The model under review builds one solid part; all positions refer to its coordinate system, in mm. Face numbers are marked on the shaded views. A direction names the side the tool comes from. Round coordinates to 2 decimals unless told otherwise and drop trailing zeros. Write each loop counter-clockwise with the first axis right and the second up, starting at its lowest first coordinate (ties: lowest second). Pieces come first, ordered by that corner, then holes.
Item 1: Draft analysis for pull direction Z (two halves, no side actions). For the marked faces 3, 4, 5 and 6, state which applies: +Z half, -Z half, draft (parallel to the pull), parting line (faces both ways), or undercut.
Item 2: Add section B-B (x = 10.5). Give the boundary of the cut face in (y, z) (3 decimals), plus the area to 3 significant figures.
Item 3: Machinability: for the marked faces 1 and 2, which of the approach directions +Z, -Z, +X, -X, +Y, -Y give a long, thin tool a straight path to every point of the face, cutting with its end or side? Answer none if there is none.
Item 4: To check wall thickness, follow L1, parallel to X at y = -3.5, z = 36.83; L2, parallel to X at y = 19.5, z = 33; L3, parallel to X at y = 8, z = 36.83. State the ranges of each line that lie inside material, in increasing order.
Item 5: Add section A-A (z = -36.83). Give the boundary of the cut face in (x, y) (3 decimals), plus the area to 3 significant figures.
Item 6: Add section D-D (y = -3.5). Give the boundary of the cut face in (x, z).
Item 7: Clearance check with flat-ended pins moving along their axes: pin 1 Ø2 at (x, z) = (28.5, 1.5) entering from +Y; pin 2 Ø8 at (x, z) = (17, 7.5) entering from -Y; pin 3 Ø5.5 at (x, y) = (-18, 8.5) entering from +Z (3 decimals); pin 4 Ø1.5 at (y, z) = (7.5, 14.5) entering from +X. State where each tip first meets the part, or that it passes through.
Item 8: Add section C-C (z = -8). State how many separate pieces and enclosed holes the cut face has, plus the area to 3 significant figures.
```python
from build123d import *

# Parameters (mm, degrees)
SKETCH1_W           = 103.124
SKETCH1_H           = 80.01
SKETCH1_W_2         = 90.424
SKETCH1_H_2         = 70.612
BOSS_EXTRUDE3_DEPTH = 21.59
SKETCH1_4_W         = 90.424
SKETCH1_4_H         = 70.612
SKETCH1_4_R         = 1.27
SKETCH1_4_W_2       = 6.35
SKETCH1_4_H_2       = 38.1
BOSS_EXTRUDE4_DEPTH = 2.54
SKETCH2_W           = 16.256
SKETCH2_H           = 14.732
SKETCH2_W_2         = 13.208
SKETCH2_H_2         = 16.51
CUT_EXTRUDE1_DEPTH  = 6.35
SKETCH6_W           = 65.024
SKETCH6_H           = 9.525
CUT_EXTRUDE2_DEPTH  = 3.048
SKETCH8_R           = 2.393
SKETCH8_R_2         = 1.25
BOSS_EXTRUDE5_DEPTH = 6.35


# Read off the part's stored shape, not the designer's step: Ø2.5mm Dowel Hole1
with BuildPart() as part:
    # Sketch1 → Boss-Extrude3 (new body)
    with BuildSketch(Plane(origin=(0, 0, 0), x_dir=(1, 0, 0), z_dir=(0, 1, 0))):
        Rectangle(SKETCH1_W, SKETCH1_H)
        with Locations((0, -1.651)):
            Rectangle(SKETCH1_W_2, SKETCH1_H_2, mode=Mode.SUBTRACT)
    extrude(amount=BOSS_EXTRUDE3_DEPTH)

    # Sketch1<4> → Boss-Extrude4 (add)
    with BuildSketch(Plane(origin=(0, 0, 0), x_dir=(1, 0, 0), z_dir=(0, 1, 0))):
        with Locations((0, -1.651)):
            Rectangle(SKETCH1_4_W, SKETCH1_4_H)
        with Locations(Location((-40.024126951, -20.193, 0), (0, 0, 270))):
            Circle(SKETCH1_4_R, mode=Mode.SUBTRACT)
        with Locations((-30.48, 0)):
            Rectangle(SKETCH1_4_W_2, SKETCH1_4_H_2, mode=Mode.SUBTRACT)
        with Locations((-15.24, 0)):
            Rectangle(SKETCH1_4_W_2, SKETCH1_4_H_2, mode=Mode.SUBTRACT)
        Rectangle(SKETCH1_4_W_2, SKETCH1_4_H_2, mode=Mode.SUBTRACT)
        with BuildLine():
            ThreePointArc((18.415, -19.037561911), (18.956131264, -19.506178054), (19.157873049, -20.193))
            ThreePointArc((19.157873049, -20.193), (16.819614834, -20.879821946), (18.415, -19.037561911))
        make_face(mode=Mode.SUBTRACT)
        Polygon((12.065, -19.05), (12.065, 19.05), (18.415, 19.05), (18.415, -13.196681286), (15.24, -13.196681286), (15.24, -19.05), align=None, mode=Mode.SUBTRACT)
        with Locations((30.48, 0)):
            Rectangle(SKETCH1_4_W_2, SKETCH1_4_H_2, mode=Mode.SUBTRACT)
        with Locations(Location((-40.024126951, 28.575, 0), (0, 0, 270))):
            Circle(SKETCH1_4_R, mode=Mode.SUBTRACT)
        with Locations(Location((17.887873049, 28.575, 0), (0, 0, 270))):
            Circle(SKETCH1_4_R, mode=Mode.SUBTRACT)
    extrude(amount=BOSS_EXTRUDE4_DEPTH)

    # Sketch2 → Cut-Extrude1 (cut)
    with BuildSketch(Plane(origin=(51.562, 0, 0), x_dir=(0, 0, -1), z_dir=(1, 0, 0))):
        with Locations((-12.827, 9.906)):
            Rectangle(SKETCH2_W, SKETCH2_H)
        with Locations((5.715, 10.795)):
            Rectangle(SKETCH2_W_2, SKETCH2_H_2)
        with Locations((23.241, 10.795)):
            Rectangle(SKETCH2_W_2, SKETCH2_H_2)
    extrude(amount=-CUT_EXTRUDE1_DEPTH, mode=Mode.SUBTRACT)

    # Ø2.5mm Dowel Hole1 outline → Ø2.5mm Dowel Hole1 (revolve, cut)
    with BuildSketch(Plane(origin=(48.387, 0, -36.83), x_dir=(1, 0, 0), z_dir=(0, 0, 1))):
        Polygon((0, 0), (1.25, 0), (1.25, 21.565), (1.275, 21.59), (0, 21.59), align=None)
    revolve(axis=Axis((48.387, 0, -36.83), (0, 1, 0)), mode=Mode.SUBTRACT)

    # 2.5mm Dowel Hole1 2 outline → 2.5mm Dowel Hole1 2 (revolve, cut)
    with BuildSketch(Plane(origin=(48.387, 0, 36.83), x_dir=(1, 0, 0), z_dir=(0, 0, 1))):
        Polygon((0, 0), (1.25, 0), (1.25, 21.565), (1.275, 21.59), (0, 21.59), align=None)
    revolve(axis=Axis((48.387, 0, 36.83), (0, 1, 0)), mode=Mode.SUBTRACT)

    # 2.5mm Dowel Hole1 3 outline → 2.5mm Dowel Hole1 3 (revolve, cut)
    with BuildSketch(Plane(origin=(-48.387, 0, -36.83), x_dir=(1, 0, 0), z_dir=(0, 0, 1))):
        Polygon((0, 0), (1.25, 0), (1.25, 21.565), (1.275, 21.59), (0, 21.59), align=None)
    revolve(axis=Axis((-48.387, 0, -36.83), (0, 1, 0)), mode=Mode.SUBTRACT)

    # 2.5mm Dowel Hole1 4 outline → 2.5mm Dowel Hole1 4 (revolve, cut)
    with BuildSketch(Plane(origin=(-48.387, 0, 36.83), x_dir=(1, 0, 0), z_dir=(0, 0, 1))):
        Polygon((0, 0), (1.25, 0), (1.25, 21.565), (1.275, 21.59), (0, 21.59), align=None)
    revolve(axis=Axis((-48.387, 0, 36.83), (0, 1, 0)), mode=Mode.SUBTRACT)

    # Sketch6 → Cut-Extrude2 (cut)
    with BuildSketch(Plane.XY.offset(40.005)):
        with Locations((-12.7, 7.9375)):
            Rectangle(SKETCH6_W, SKETCH6_H)
    extrude(amount=-CUT_EXTRUDE2_DEPTH, mode=Mode.SUBTRACT)

    # Sketch8 → Boss-Extrude5 (add)
    # profile 1 of 4: a face of its own
    with BuildSketch(Plane.XZ):
        with Locations(Location((-48.387, 36.83, 0), (0, 0, 90))):
            Circle(SKETCH8_R)
        with Locations(Location((-48.387, 36.83, 0), (0, 0, 90))):
            Circle(SKETCH8_R_2, mode=Mode.SUBTRACT)
    # profile 2 of 4: a face of its own
    with BuildSketch(Plane.XZ):
        with Locations(Location((48.387, 36.83, 0), (0, 0, 270))):
            Circle(SKETCH8_R)
        with Locations(Location((48.387, 36.83, 0), (0, 0, 90))):
            Circle(SKETCH8_R_2, mode=Mode.SUBTRACT)
    # profile 3 of 4: a face of its own
    with BuildSketch(Plane.XZ):
        with Locations(Location((48.387, -36.83, 0), (0, 0, 90))):
            Circle(SKETCH8_R)
        with Locations(Location((48.387, -36.83, 0), (0, 0, 90))):
            Circle(SKETCH8_R_2, mode=Mode.SUBTRACT)
    # profile 4 of 4: a face of its own
    with BuildSketch(Plane.XZ):
        with Locations(Location((-48.387, -36.83, 0), (0, 0, 270))):
            Circle(SKETCH8_R)
        with Locations(Location((-48.387, -36.83, 0), (0, 0, 90))):
            Circle(SKETCH8_R_2, mode=Mode.SUBTRACT)
    extrude(amount=BOSS_EXTRUDE5_DEPTH)


solid = part.part
```
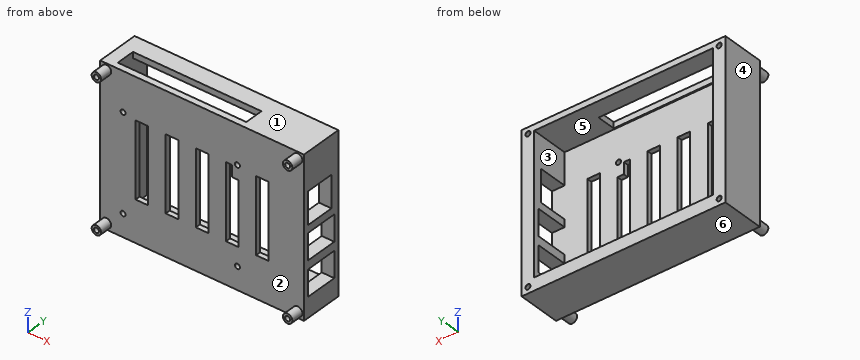
Numbers:
1. face 3: undercut
1. face 4: draft
1. face 5: undercut
1. face 6: -Z half
2. outline: (0, -40.005) - (21.59, -40.005) - (21.59, -33.655) - (2.54, -33.655) - (2.54, 36.957) - (3.175, 36.957) - (3.175, 40.005) - (0, 40.005) - close; (12.7, 36.957) - (21.59, 36.957) - (21.59, 40.005) - (12.7, 40.005) - close
2. area: 353 mm2
3. face 1: +Z, +X, -X, +Y, -Y
3. face 2: -Y
4. L1: x = -50.78 to -49.64, -47.14 to -45.99, 45.99 to 47.14, 49.64 to 50.78
4. L2: x = -51.56 to -45.21, 45.21 to 51.56
4. L3: x = -51.56 to -49.64, -47.14 to -45.21, 45.21 to 47.14, 49.64 to 51.56
5. outline: (-51.562, 0) - (-50.78, 0) - (-50.78, -6.35) - (-49.637, -6.35) - (-49.637, 21.565) - (-49.662, 21.59) - (-51.562, 21.59) - close; (-47.137, -6.35) - (-45.994, -6.35) - (-45.994, 0) - (45.994, 0) - (45.994, -6.35) - (47.137, -6.35) - (47.137, 21.565) - (47.112, 21.59) - (-47.112, 21.59) - (-47.137, 21.565) - close; (49.637, -6.35) - (50.78, -6.35) - (50.78, 0) - (51.562, 0) - (51.562, 21.59) - (49.662, 21.59) - (49.637, 21.565) - close
5. area: 2,150 mm2
6. outline: circle Ø4.79 at (-48.39, -36.83); circle Ø4.79 at (-48.39, 36.83); circle Ø4.79 at (48.39, -36.83); circle Ø4.79 at (48.39, 36.83); hole circle Ø2.5 at (-48.39, -36.83); hole circle Ø2.5 at (-48.39, 36.83); hole circle Ø2.5 at (48.39, -36.83); hole circle Ø2.5 at (48.39, 36.83)
7. pin 1: passes through
7. pin 2: stops at y = 0
7. pin 3: stops at z = -33.655
7. pin 4: stops at x = -45.21
8. separate pieces: 7
8. enclosed holes: 0
8. area: 318 mm2
